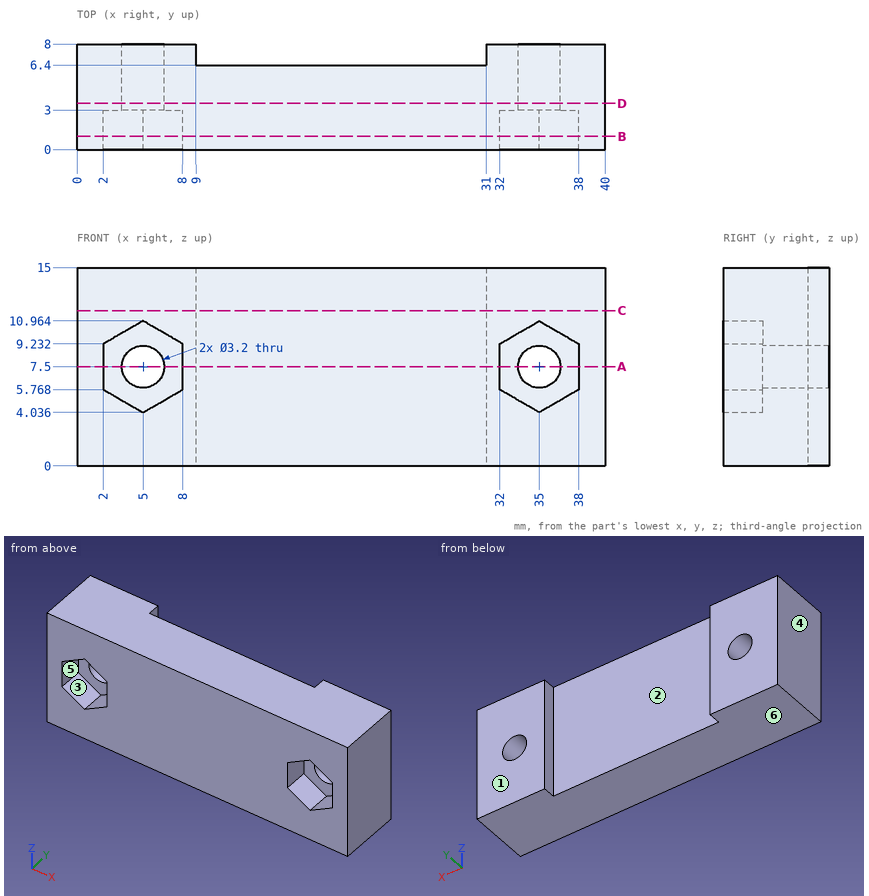
Here's the drawing with two shaded views (mm, measured from the low corner). I have some questions. A direction names the side the tool comes from. Give positions to 0.01 mm unless a question says otherwise; leave off trailing zeros. Loops run counter-clockwise (first coordinate to the right, second up) from the corner with the lowest first, then second, coordinate; pieces in that order, holes last. Notation, with made-up numbers: M 87,65 L 93,65 A31 ccw 93,100 Z; hole C 35.25,45.5 d1. An arc over 180 degrees is marked long. Answer in a Markdown table with one row per item.
1. Suppose I cut it at C-C on z = 11.75. Write out the boundary of the cut face in (x, y).
Taken from the geometry:
| item | result |
|---|---|
| outline | M 0,0 L 40,0 L 40,8 L 31,8 L 31,6.4 L 9,6.4 L 9,8 L 0,8 Z |
2. Thinking about a two-plate mould opening in Z: for the marked faces 4, 5 and 6, which applies, released by +Z, released by -Z, zero draft, split by the parting line, or undercut?
Taken from the geometry:
| item | result |
|---|---|
| face 4 | zero draft |
| face 5 | undercut |
| face 6 | released by -Z |
3. Suppose I cut it at B-B on y = 1. Write out the boundary of the cut face in (x, z), plus the area to 3 significant figures.
Taken from the geometry:
| item | result |
|---|---|
| outline | M 0,0 L 40,0 L 40,15 L 0,15 Z; hole M 2,5.77 L 5,4.04 L 8,5.77 L 8,9.23 L 5,10.96 L 2,9.23 Z; hole M 32,5.77 L 35,4.04 L 38,5.77 L 38,9.23 L 35,10.96 L 32,9.23 Z |
| area | 538 mm² |
4. Which directions (+Z, -Z, +X, -X, +Y, -Y) give clear straight access to the entire face, cutting with the end or side of a thin tool? Please do the marked faces 1, 2 and 3.
Taken from the geometry:
| item | result |
|---|---|
| face 1 | +Z, -Z, +X, -X, +Y |
| face 2 | +Z, -Z, +Y |
| face 3 | -Y |
5. Suppose I cut it at A-A on z = 7.5. Write out the boundary of the cut face in (x, y).
Taken from the geometry:
| item | result |
|---|---|
| outline | M 0,0 L 2,0 L 2,3 L 3.4,3 L 3.4,8 L 0,8 Z; M 6.6,3 L 8,3 L 8,0 L 32,0 L 32,3 L 33.4,3 L 33.4,8 L 31,8 L 31,6.4 L 9,6.4 L 9,8 L 6.6,8 Z; M 36.6,3 L 38,3 L 38,0 L 40,0 L 40,8 L 36.6,8 Z |
6. If I drill on line 1 along X through (y, z) = (2, 6.5); line 2 along X through (y, z) = (4.9, 7.5); line 3 along X through (y, z) = (7.5, 4), over which ranges is the centre line in solid material (lowest first)?
Taken from the geometry:
| item | result |
|---|---|
| line 1 | x = 0 to 2, 8 to 32, 38 to 40 |
| line 2 | x = 0 to 3.4, 6.6 to 33.4, 36.6 to 40 |
| line 3 | x = 0 to 9, 31 to 40 |
7. For pin 1 Ø1.3 at (y, z) = (7.5, 5) entering from -X; pin 2 Ø3 at (x, z) = (35, 7.5) entering from -Y; pin 3 Ø3.5 at (x, z) = (5, 7.5) entering from -Y, each with a flat end and sliding along its axis, tell me the tip position at first contact or that it passes through.
Taken from the geometry:
| item | result |
|---|---|
| pin 1 | stops at x = 0 |
| pin 2 | passes through |
| pin 3 | stops at y = 3 |
8. Suppose I cut it at D-D on y = 3.5. Write out the boundary of the cut face in (x, z), plus the area to 3 significant figures.
Taken from the geometry:
| item | result |
|---|---|
| outline | M 0,0 L 40,0 L 40,15 L 0,15 Z; hole C 5,7.5 d3.2; hole C 35,7.5 d3.2 |
| area | 584 mm² |
